Work out the finished part from the listing and answer in its coordinate system (mm). A direction names the side the tool comes from. Give positions to 0.01 mm unless a question says otherwise; leave off trailing zeros. Order: outer loops, then holes, each group sorted by start corner. A loop starts at its lowest first (then second) coordinate and runs counter-clockwise, first axis right, second up. Notation, with made-up numbers: (-29, 34) -> (24, 34) arc R19 cw to (24, 53) -> close; hole circle Ø4 at (65.5, 80.25). An arc over 180 degrees is marked (long way). Use a Markdown table: item, result. Add a question column.
```python
from build123d import *

# Parameters (mm, degrees)
EXTRUDE1_DEPTH = 167
EXTRUDE2_DEPTH = 125
EXTRUDE3_DEPTH = 77
SKETCH10_R     = 15
EXTRUDE4_DEPTH = 1


with BuildPart() as part:
    # Sketch1 → Revolve1 (revolve)
    with BuildSketch(Plane.XY, mode=Mode.PRIVATE) as revolve1_sk:
        Polygon((0, 113), (-30, 113), (-30, 108), (-83, 108), (-83, 57.5), (-250, 57.5), (-250, 150), (0, 150), align=None)
    revolve(revolve1_sk.sketch.rotate(Axis((0, 0, 0), (1, 0, 0)), 90), axis=Axis((0, 0, 0), (1, 0, 0)))

    # Sketch2 → Extrude1 (cut)
    with BuildSketch(Plane.ZY.offset(250)):
        with BuildLine():
            Line((13.8, -55.819441058), (108.04, -32.520891747))
            ThreePointArc((108.04, -32.520891747), (133.5, 0), (108.04, 32.520891747))
            Line((108.04, 32.520891747), (13.8, 55.819441058))
            ThreePointArc((13.8, 55.819441058), (57.5, 0), (13.8, -55.819441058))
        make_face()
    extrude(amount=-EXTRUDE1_DEPTH, mode=Mode.SUBTRACT)

    # Sketch5 → Cut-Revolve1 (revolve, cut)
    with BuildSketch(Plane.XY, mode=Mode.PRIVATE) as cut_revolve1_sk:
        Polygon((-125, 135.5), (-262.537169633, 135.5), (-262.537169633, 100), (-106, 100), (-106, 125), (-108, 125), (-108, 127.5), (-121, 127.5), (-121, 128.5), (-122, 128.5), (-122, 127.5), (-125, 127.5), align=None)
    revolve(cut_revolve1_sk.sketch.rotate(Axis((-262.537169633, 100, 0), (1, 0, 0)), 90), axis=Axis((-262.537169633, 100, 0), (1, 0, 0)), mode=Mode.SUBTRACT)

    # Sketch6 → Extrude2 (cut)
    with BuildSketch(Plane.ZY.offset(250)):
        with BuildLine():
            Line((-34.630245451, 107.81), (-56.091242632, 12.65))
            ThreePointArc((-56.091242632, 12.65), (0, -57.5), (56.091242632, 12.65))
            Line((56.091242632, 12.65), (34.630245451, 107.81))
            ThreePointArc((34.630245451, 107.81), (0, 135.5), (-34.630245451, 107.81))
        make_face()
    extrude(amount=-EXTRUDE2_DEPTH, mode=Mode.SUBTRACT)

    # Sketch7 → Cut-Revolve2 (revolve, cut)
    with BuildSketch(Plane(origin=(0, 0, 0), x_dir=(1, 0, 0), z_dir=(0, 1, 0))):
        Polygon((-250, 135.5), (-173, 135.5), (-173, 127.5), (-170, 127.5), (-170, 128.5), (-169, 128.5), (-169, 127.5), (-156, 127.5), (-156, 125), (-154, 125), (-154, 100), (-250, 100), align=None)
    revolve(axis=Axis((-154, 0, -100), (-1, 0, 0)), mode=Mode.SUBTRACT)

    # Sketch8 → Extrude3 (cut)
    with BuildSketch(Plane.ZY.offset(250)):
        with BuildLine():
            Line((-107.81, 34.630245451), (-12.65, 56.091242632))
            ThreePointArc((-12.65, 56.091242632), (57.5, 0), (-12.65, -56.091242632))
            Line((-12.65, -56.091242632), (-107.81, -34.630245451))
            ThreePointArc((-107.81, -34.630245451), (-135.5, 0), (-107.81, 34.630245451))
        make_face()
    extrude(amount=-EXTRUDE3_DEPTH, mode=Mode.SUBTRACT)

    # Sketch10 → Extrude4 (cut)
    with BuildSketch(Plane(origin=(0, -150, 0), x_dir=(-1, 0, 0), z_dir=(0, -1, 0))):
        with Locations(Location((125, 0, 0), (0, 0, 90))):
            Circle(SKETCH10_R)
    extrude(amount=-EXTRUDE4_DEPTH, mode=Mode.SUBTRACT)


solid = part.part
```
1) The part is cut by section D-D, the plane x = -223. Determine the outline of the cut face in (y, z).
2) Which of the six approach directions +Z, -Z, +X, -X, +Y, -Y give full straight-line access (tool end or side, diameter ignored) to faces 1 (the flat face through (0, -112, 22)), 2 (the flat face through (-156, 22.3, -112.1)), 3 (the cylindrical face through (-123.25, 133.076, 69.216)), 4 (the cylindrical face through (-114.862, -149.396, 11.056)), 5 (the cylindrical face through (-15.21, -95.28, 60.75))?
3) Determine the mould class of faces 6 (the cylindrical face through (-169.493, -1.253, -71.528)), 7 (the flat face through (-173, 0, -69)), 8 (the flat face through (-169, -23.4, -85.1)), 9 (the flat face through (-83, 46, -51)) for opening direction X: released by +X, released by -X, zero draft, split by the parting line, or undercut.
4) Flat-ended cylindrical pins translate along their axes: pin 1 (1 mm diameter, centred on x = -106.5, z = -84, fed in from -Y); pin 2 (4 mm diameter, centred on x = -139.5, z = 53.5, fed in from -Y); pin 3 (10 mm diameter, centred on x = -43, z = 78.5, fed in from -Y). Find the tip coordinate at first contact, or state that the pin passes through.
5) Straight lines are drawn through the part: line 1 (Y direction, x = -58, z = 0); line 2 (Y direction, x = -7.5, z = 0); line 3 (Z direction, x = -54, y = 66). For each, find the intervals that lie inside material, in ascending order.
6) The part is cut by section B-B, the plane x = -163.5. Determine the outline of the cut face in (y, z), then the cut area to 3 significant figures.
7) The part is cut by section C-C, the plane z = 88. Determine the outline of the cut face in (x, y), then the cut area to 3 significant figures.
A:
| question | item | result |
|---|---|---|
| 1 | outline | circle Ø300 at (0, 0); hole (-56.09, -12.65) -> (-34.63, -107.81) arc R35.5 ccw to (34.63, -107.81) -> (48.1, -48.1) -> (107.81, -34.63) arc R35.5 ccw to (107.81, 34.63) -> (47.3, 48.28) -> (32.52, 108.04) arc R33.5 ccw to (-32.52, 108.04) -> (-55.82, 13.8) arc R57.5 ccw to start |
| 2 | face 1 | +Z, -Z, +X, +Y, -Y |
| 2 | face 2 | -X |
| 2 | face 3 | +X, -X |
| 2 | face 4 | -Y |
| 2 | face 5 | +X |
| 3 | face 6 | undercut |
| 3 | face 7 | released by -X |
| 3 | face 8 | undercut |
| 3 | face 9 | released by +X |
| 4 | pin 1 | y = -124.61 |
| 4 | pin 2 | y = -140.88 |
| 4 | pin 3 | y = -130.76 |
| 5 | line 1 | -150 to -108, 108 to 150 |
| 5 | line 2 | -150 to -113, 113 to 150 |
| 5 | line 3 | -134.7 to -85.49, 85.49 to 134.7 |
| 6 | outline | circle Ø300 at (0, 0); hole (-55.82, 13.8) arc R57.5 ccw to (12.65, -56.09) -> (107.81, -34.63) arc R35.5 ccw to (107.81, 34.63) -> (47.3, 48.28) -> (32.52, 108.04) arc R33.5 ccw to (-32.52, 108.04) -> close; hole circle Ø55 at (0, -100) |
| 6 | area | 45,900 mm^2 |
| 7 | outline | (-250, -121.47) -> (0, -121.47) -> (0, -70.89) -> (-30, -70.89) -> (-30, -62.61) -> (-83, -62.61) -> (-83, -37.48) -> (-250, -37.48) -> close; (-250, 37.48) -> (-83, 37.48) -> (-83, 62.61) -> (-30, 62.61) -> (-30, 70.89) -> (0, 70.89) -> (0, 121.47) -> (-250, 121.47) -> close |
| 7 | area | 37,300 mm^2 |
